Source: CAD feature listing. Evaluate the final solid. Frame: model axes, mm. Face numbers are marked on the shaded views. A direction names the side the tool comes from. Coordinates: 2 decimals unless noted, no trailing zeros. Loops run counter-clockwise (first coordinate to the right, second up) from the corner with the lowest first, then second, coordinate; pieces in that order, holes last. Notation, with made-up numbers: (47.5, 66.25) - (85.5, 66.25) arc R19 cw to (85.5, 102.25) - close; hole circle Ø1 at (83.5, 41). An arc over 180 degrees is marked (long way). Use one line per item in the form item = value. Start each with the question number.
from build123d import *

# Parameters (mm, degrees)
F0_R     = 50
F0_R_2   = 40
F1_DEPTH = 85
F4_DEPTH = 16
F6_DEPTH = 18
F8_DEPTH = 17
F9_SIZE  = 9.99999


# Not quite as in the source:
# - a fillet or chamfer is up to 0.001 mm smaller than in the source, because OpenCascade refuses the exact size
# - a feature names something its author has since deleted; it is built from what else it names


with BuildPart() as f1:
    # F0 (on Front) → F1 (new body)
    with BuildSketch(Plane.XZ):
        Circle(F0_R)
        Circle(F0_R_2, mode=Mode.SUBTRACT)
    extrude(amount=F1_DEPTH)

    # F3 (on offset) → F4 (join)
    with BuildSketch(Plane.XZ.offset(9)):
        with BuildLine():
            ThreePointArc((-48.0294117647, -13.898762734), (-39.9683508335, 30.0421525802), (0, 50))
            Line((0, 50), (0, 100))
            ThreePointArc((0, 100), (-75.4648138983, 65.6129702368), (-99.0294117647, -13.898762734))
            Line((-99.0294117647, -13.898762734), (-48.0294117647, -13.898762734))
        make_face()
    extrude(amount=F4_DEPTH)

    # F5 (on offset) → F6 (cut)
    with BuildSketch(Plane.XZ.offset(9)):
        with BuildLine():
            ThreePointArc((-24, 80), (-34.9315537053, 83.4175690266), (-27.8932593505, 74.3820249346))
            ThreePointArc((-27.8932593505, 74.3820249346), (-25.0684462947, 76.5824309734), (-24, 80))
        make_face()
        with BuildLine():
            ThreePointArc((-79, 10), (-90.989717095, 10.3511255077), (-79.0410963741, 9.2989525146))
            ThreePointArc((-79.0410963741, 9.2989525146), (-79.010282905, 9.6488744923), (-79, 10))
        make_face()
    extrude(amount=F6_DEPTH, mode=Mode.SUBTRACT)

    # F7 (on face) → F8 (cut)
    with BuildSketch(Plane.XZ.offset(25)):
        with BuildLine():
            ThreePointArc((-75.732676721, 21.7947750823), (-40.5874083787, 31.7115351547), (-39.267323279, 68.2052249177))
            ThreePointArc((-39.267323279, 68.2052249177), (-44.9963531804, 80.3307435394), (-38.7382990756, 92.1918878466))
            ThreePointArc((-38.7382990756, 92.1918878466), (-78.5370863203, 61.9025530355), (-98.6907067749, 16.1289924134))
            ThreePointArc((-98.6907067749, 16.1289924134), (-88.5940024625, 24.5630747543), (-75.732676721, 21.7947750823))
        make_face()
    extrude(amount=-F8_DEPTH, mode=Mode.SUBTRACT)

    # F9 (size 10 in the source; OpenCascade refuses exactly that, so slightly less here)
    f9_edges = [f1.edges().sort_by_distance(p)[0] for p in [
        (-50, -85, 0),
    ]]
    chamfer(f9_edges, length=F9_SIZE)


solid = f1.part
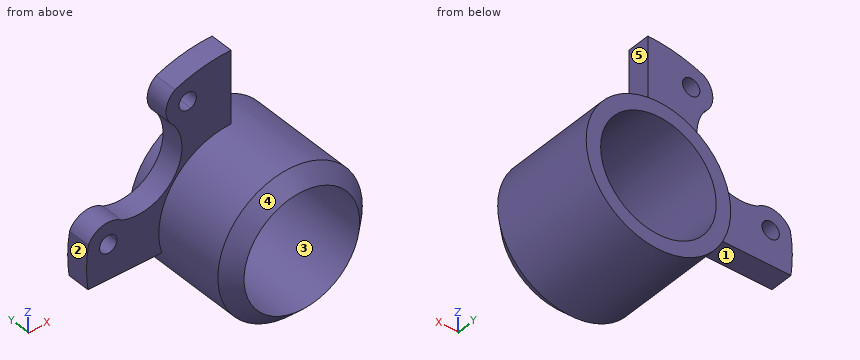
(1) Cut plane C-C, the plane y = -77.5. Output: boundary loops of the cut face in (x, z), plus the area to 3 significant figures.
(2) Cut plane A-A, the plane x = -85. Output: boundary loops of the cut face in (y, z).
(3) Contact query for flat-ended pins moving along their axis: pin 1 (5 mm diameter, centred on x = 28.5, y = -39.5, fed in from -Z); pin 2 (8 mm diameter, centred on y = -59.5, z = 5, fed in from -X); pin 3 (8 mm diameter, centred on x = -6, z = 79.5, fed in from -Y); pin 4 (9.5 mm diameter, centred on x = -85, z = 10, fed in from -Y). Output: stop coordinate, or through.
(4) Access query for the marked faces 4 and 5. Directions: +Z, -Z, +X, -X, +Y, -Y. A direction counts if a zero-diameter tool reaches every point of the face in a straight line with its end or side. Return the directions, or none.
(5) Mould query, pull axis X, two halves, no side actions, for the marked faces 1, 2 and 3. Classes: +X half, -X half, draft (parallel to the pull), parting line (faces both ways), or undercut.
(6) Material intervals for line 1 (X direction, y = -19.75, z = 80); line 2 (Z direction, x = -30, y = -16.25); line 3 (Z direction, x = 9.5, y = -8), sorted ascending.
(7) Cut plane D-D, the plane y = -19. Output: boundary loops of the cut face in (x, z), plus the area to 3 significant figures.
Recorded:
q1.outline = circle Ø95 at (0, 0); hole circle Ø80 at (0, 0)
q1.area = 2,060 mm²
q2.outline = (-25, -13.9) - (-9, -13.9) - (-9, 4) - (-25, 4) - close; (-25, 16) - (-9, 16) - (-9, 25) - (-25, 25) - close
q3.pin_1 = -42.71
q3.pin_2 = -49.99
q3.pin_3 = -25
q3.pin_4 = through
q4.face_4 = -Y
q4.face_5 = +Z, +X, +Y, -Y
q5.face_1 = draft
q5.face_2 = -X half
q5.face_3 = undercut
q6.line_1 = -45 to -36, -24 to 0
q6.line_2 = -40 to -26.46, 26.46 to 74, 86 to 95.39
q6.line_3 = -49.09 to -38.86, 38.86 to 49.09
q7.outline = (-99.03, -13.9) - (-48.03, -13.9) arc R50 ccw (long way) to (0, 50) - (0, 100) arc R100 ccw to (-38.74, 92.19) arc R15 ccw to (-39.27, 68.21) arc R31 cw to (-75.73, 21.79) arc R15 ccw to (-98.69, 16.13) arc R100 ccw to start; hole circle Ø12 at (-85, 10); hole circle Ø80 at (0, 0); hole circle Ø12 at (-30, 80)
q7.area = 6,510 mm²
